from build123d import *

# Parameters (mm, degrees)
SKETCH_1_W          = 5.08
SKETCH_1_H          = 2.54
EXTRUDE_1_DEPTH     = 14.1
SKETCH_5_W          = 0.8
SKETCH_5_H          = 0.8
CUT_EXTRUDE_5_DEPTH = 10
CHAMFER_5_SIZE      = 0.4
SKETCH_2_W          = 0.8
SKETCH_2_H          = 0.8
CUT_EXTRUDE_2_DEPTH = 10


with BuildPart() as part:
    # Эскиз1 → Бобышка-Вытянуть1 (new body)
    with BuildSketch(Plane(origin=(0, 0, 0), x_dir=(1, 0, 0), z_dir=(0, 1, 0))):
        with Locations((2.54, 1.27)):
            Rectangle(SKETCH_1_W, SKETCH_1_H)
    extrude(amount=EXTRUDE_1_DEPTH)

    # Эскиз5 → Вырез-Вытянуть5 (cut)
    with BuildSketch(Plane(origin=(0, 14.1, 0), x_dir=(1, 0, 0), z_dir=(0, 1, 0))):
        with Locations((1.27, 1.27)):
            Rectangle(SKETCH_5_W, SKETCH_5_H)
        with Locations((3.79891982, 1.27)):
            Rectangle(SKETCH_5_W, SKETCH_5_H)
    extrude(amount=-CUT_EXTRUDE_5_DEPTH, mode=Mode.SUBTRACT)

    # Фаска5
    chamfer_5_edges = [part.edges().sort_by_distance(p)[0] for p in [
        (0.87, 14.1, -1.27),
        (1.27, 14.1, -1.67),
        (1.27, 14.1, -0.87),
        (1.67, 14.1, -1.27),
        (3.39891982, 14.1, -1.27),
        (3.79891982, 14.1, -1.67),
        (3.79891982, 14.1, -0.87),
        (4.19891982, 14.1, -1.27),
    ]]
    chamfer(chamfer_5_edges, length=CHAMFER_5_SIZE)

    # Эскиз2 → Вырез-Вытянуть2 (cut)
    with BuildSketch(Plane(origin=(0, 14.1, 0), x_dir=(1, 0, 0), z_dir=(0, 1, 0))):
        with Locations((1.27, 1.27)):
            Rectangle(SKETCH_2_W, SKETCH_2_H)
        with Locations((3.81, 1.27)):
            Rectangle(SKETCH_2_W, SKETCH_2_H)
    extrude(amount=-CUT_EXTRUDE_2_DEPTH, mode=Mode.SUBTRACT)


solid = part.part
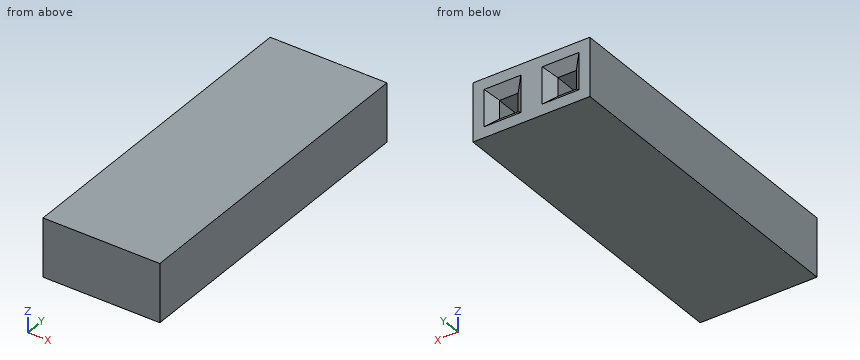
Geometry check sheet. Reference: the model listing, model coordinates, mm. Round coordinates to 2 decimals unless told otherwise and drop trailing zeros. Write each loop counter-clockwise with the first axis right and the second up, starting at its lowest first coordinate (ties: lowest second). Pieces come first, ordered by that corner, then holes.
Item 1: Go/stop test with a flat-tipped pin: pin 1 Ø3 at (x, y) = (3.5, 2) entering from +Z. Record where the tip stops, or that it passes through.
Determined:
pin 1: stops at z = 0
Item 2: Section check A-A (x = 1). Record the boundary of the cut face in (y, z), plus the area to 3 significant figures.
Determined:
outline: (0, -2.54) - (14.1, -2.54) - (14.1, -2.07) - (13.7, -1.67) - (4.1, -1.67) - (4.1, -0.87) - (13.7, -0.87) - (14.1, -0.47) - (14.1, 0) - (0, 0) - close
area: 27.7 mm2
Item 3: Section check C-C (z = -1.4). Record the boundary of the cut face in (x, y), plus the area to 3 significant figures.
Determined:
outline: (0, 0) - (5.08, 0) - (5.08, 14.1) - (4.6, 14.1) - (4.21, 13.71) - (4.21, 4.1) - (3.4, 4.1) - (3.4, 13.7) - (3, 14.1) - (2.07, 14.1) - (1.67, 13.7) - (1.67, 4.1) - (0.87, 4.1) - (0.87, 13.7) - (0.47, 14.1) - (0, 14.1) - close
area: 55.2 mm2
Item 4: Material ranges on line 1 along X through (y, z) = (9.5, -1.2); line 2 along Z through (x, y) = (3.8, 5.25); line 3 along Y through (x, z) = (3.2, -1.9), recorded low to high.
Determined:
line 1: x = 0 to 0.87, 1.67 to 3.4, 4.21 to 5.08
line 2: z = -2.54 to -1.67, -0.87 to 0
line 3: y = 0 to 13.93
Item 5: Section check B-B (y = 11). Record the boundary of the cut face in (x, z).
Determined:
outline: (0, -2.54) - (5.08, -2.54) - (5.08, 0) - (0, 0) - close; hole (0.87, -1.67) - (1.67, -1.67) - (1.67, -0.87) - (0.87, -0.87) - close; hole (3.4, -1.67) - (4.21, -1.67) - (4.21, -0.87) - (3.4, -0.87) - close
